Autodesk Inventor part; units mm, degrees
ref_plane "YZ Plane" through (0, 0, 0) normal (1, 0, 0) x (0, 1, 0)
ref_plane "XZ Plane" through (0, 0, 0) normal (0, 1, 0) x (-1, 0, 0)
ref_plane "XY Plane" through (0, 0, 0) normal (0, 0, 1) x (1, 0, 0)
sketch "Sketch1" plane through (0, 0, 0) normal (1, 0, 0) x (0, 1, 0)
  circle A0 centre (0, 0) radius 1.5
  line L0 (0, 0) -> (0, -30)
  circle A1 centre (0, -30) radius 1.5
  arc A2 (-4.5, -30) -> (0, -25.5) centre (0, -30) ccw
  arc A3 (4.5, 0) -> (0, -4.5) centre (0, 0) ccw
  line L1 (4.5, 0) -> (4.5, -30)
  line L2 (-4.5, 0) -> (-4.5, -30)
  line L3 (4.5, 0) -> (4.5, -15)
  line L4 (4.5, -15) -> (4.5, -19)
  line L5 (4.5, -15) -> (4.5, -11)
  line L6 (4.5, -11) -> (9.5, -11)
  line L7 (4.5, -19) -> (9.5, -19)
  line L8 (9.5, -11) -> (9.5, -19)
  line L9 (9.5, -19) -> (9.5, -15)
  line L10 (9.5, -15) -> (14, -15)
  line L11 (14, -15) -> (14, -65)
  line L12 (0, 0) -> (14, 14.2829)
  circle A4 centre (14, 14.2829) radius 1.5
  circle A5 centre (14, 14.2829) radius 4.5
  line L13 (14, -15) -> (14, 15.7829)
  line L14 (14, 18.7829) -> (14, 35)
  line L15 (9.5, 14.2829) -> (9.5, -11)
  line L16 (0, -30) -> (14, -41.3137)
  circle A6 centre (14, -41.3137) radius 1.5
  circle A7 centre (14, -41.3137) radius 4.5
  line L17 (9.5, -19) -> (9.5, -41.3137)
  line L18 (18.5, -41.3137) -> (18.5, 14.2829)
  dimension "d15" = 3
  dimension "d0" = 3
  dimension "d1" = 30
  dimension "d2" = 3
  dimension "d3" = 9
  dimension "d4" = 9
  dimension "d5" = 15
  dimension "d6" = 4
  dimension "d7" = 4
  dimension "d8" = 5
  dimension "d9" = 5
  dimension "d10" = 4
  dimension "d11" = 4.5
  dimension "d12" = 50
  dimension "d13" = 50
  dimension "d14" = 20
  dimension "d16" = 9
  dimension "d17" = 18
  dimension "d18" = 3
  dimension "d19" = 9
extrude "Extrusion1" add sketch "Sketch1" along normal blind 2.5 contours A0 L12 A3 L1 A2 L0 | A0 L0 A3 L12 | L0 A1 L16 A2 L2 A3 | L15 A5 L12 | L12 A5 L13 L10 L8 L15 | A2 L16 A1 L0 | L6 L8 L7 L1 | A5 L13 A4 L12 | L12 A4 L13 A5 | A5 L18 A7 L11 L13 | L10 L11 A7 L16 L17 L8 | L16 A7 L17 | A7 L11 A6 L16 | L16 A6 L11 A7 | A7 L11 A6
properties part number "acople_acr"
CAD build for the part. Positions are in the model's coordinates, mm. A direction names the side the tool comes from. Coordinates: 2 decimals unless noted, no trailing zeros. Order: outer loops, then holes, each group sorted by start corner. A loop starts at its lowest first (then second) coordinate and runs counter-clockwise, first axis right, second up. Notation, with made-up numbers: M 27.5,-25.5 L 77.5,-25.5 A11 ccw 77.5,-6.5 Z; hole C 12,60 d4. An arc over 180 degrees is marked long. Write each question's results on one line, items separated by ' | '. Start each with the question number.
Q1. Cut at D-D (y = 14). List the corners of the cut face in (x, z).
Q2. Drill centre lines: probe 1 along Z at (x, y) = (0.5, 0); probe 2 along Y at (x, z) = (1.95, 0); probe 3 along Z at (x, y) = (1, 14). Where is each one in solid material? Low to high. Write a range as from..to.
Q3. Flat gauge pins, fed straight in: P1, Ø0.8, axis at x = 0.5, y = 6.5, coming from the +Z side; P2, Ø1.2, axis at x = 2, z = 7, coming from the -Y side. Where does each tip first touch, or does it go through?
Q4. Pull direction Y, two halves, no side cores. Call faces 1 (the flat face through (0, 9, -13)), 2 (the flat face through (1, 18.5, -14)), 3 (the flat face through (1, 9.5, 2)): +Y half, -Y half, draft (parallel to the pull), parting line (faces both ways), or undercut.
Q5. Which spindle directions (+Z, -Z, +X, -X, +Y, -Y) get a long thin tool onto all of the face, cutting with end or side? Do faces 4 (the flat face through (1, 7, -11)), 5 (the flat face through (1, 4.5, -24)), 6 (the cylindrical face through (1.23, 12.81, -40.4)). Say none if no direction does.
Q6. Cut at B-B (z = -27.5). List the corners of the cut face in (x, y).
Q7. Cut at C-C (x = 0.55). List the corners of the cut face in (y, z), then the cut area to 3 significant figures.
Q8. Cut at A-A (y = 0). List the corners of the cut face in (x, z), then the cut area to 3 significant figures.
Found:
1) outline: M 0,-45.81 L 2.5,-45.81 L 2.5,-42.81 L 0,-42.81 Z; M 0,-39.81 L 2.5,-39.81 L 2.5,12.78 L 0,12.78 Z; M 0,15.78 L 2.5,15.78 L 2.5,18.78 L 0,18.78 Z
2) probe 1: -34.5..-31.5, -28.5..-1.5, 1.5..4.5 | probe 2: -4.5..-1.5, 1.5..4.5, 9.5..18.5 | probe 3: -45.81..-42.81, -39.81..12.78, 15.78..18.78
3) P1: z = -11 | P2: y = 9.5
4) face 1: draft | face 2: +Y half | face 3: undercut
5) face 4: +Z, +X, -X | face 5: -Z, +X, -X | face 6: +X, -X
6) outline: M 0,-4.5 L 2.5,-4.5 L 2.5,4.5 L 0,4.5 Z; M 0,9.5 L 2.5,9.5 L 2.5,18.5 L 0,18.5 Z
7) outline: M -4.5,-30 A4.5 ccw 4.5,-30 L 4.5,-19 L 9.5,-19 L 9.5,-41.31 A4.5 ccw 18.5,-41.31 L 18.5,14.28 A4.5 ccw 9.5,14.28 L 9.5,-11 L 4.5,-11 L 4.5,0 A4.5 ccw -4.5,0 Z; hole C 0,-30 d3; hole C 0,0 d3; hole C 14,-41.31 d3; hole C 14,14.28 d3 | area: 909 mm²
8) outline: M 0,-34.5 L 2.5,-34.5 L 2.5,-31.5 L 0,-31.5 Z; M 0,-28.5 L 2.5,-28.5 L 2.5,-1.5 L 0,-1.5 Z; M 0,1.5 L 2.5,1.5 L 2.5,4.5 L 0,4.5 Z | area: 82.5 mm²
